Can you work these out from the model? Positions are in its coordinate system, mm. Face numbers are marked on the shaded views. A direction names the side the tool comes from. Round coordinates to 2 decimals unless told otherwise and drop trailing zeros. Loops run counter-clockwise (first coordinate to the right, second up) from the corner with the lowest first, then second, coordinate; pieces in that order, holes last. Notation, with made-up numbers: M 4,12 L 8,12 A13 ccw 8,24 Z; hole C 65.25,-26.5 d8. An arc over 180 degrees is marked long. Return JSON: item names as keys, results as strings.
```python
from build123d import *

# Parameters (mm, degrees)
SKETCH1_W           = 28.2
SKETCH1_H           = 28.2
SKETCH1_R           = 1.25
SKETCH1_R_2         = 10
BOSS_EXTRUDE1_DEPTH = 5
SKETCH1_3_R         = 11
SKETCH1_3_R_2       = 10
BOSS_EXTRUDE2_DEPTH = 14
SKETCH1_4_R         = 11
SKETCH1_4_R_2       = 10
CUT_EXTRUDE1_DEPTH  = 2


with BuildPart() as part:
    # Sketch1 → Boss-Extrude1 (new body)
    with BuildSketch(Plane.XY):
        Rectangle(SKETCH1_W, SKETCH1_H)
        with Locations((-11.5, 11.5)):
            Circle(SKETCH1_R, mode=Mode.SUBTRACT)
        with Locations((11.5, 11.5)):
            Circle(SKETCH1_R, mode=Mode.SUBTRACT)
        with Locations((11.5, -11.5)):
            Circle(SKETCH1_R, mode=Mode.SUBTRACT)
        with Locations((-11.5, -11.5)):
            Circle(SKETCH1_R, mode=Mode.SUBTRACT)
        Circle(SKETCH1_R_2, mode=Mode.SUBTRACT)
    extrude(amount=BOSS_EXTRUDE1_DEPTH)

    # Sketch1_3 → Boss-Extrude2 (add)
    # profile 1 of 3: a face of its own
    with BuildSketch(Plane.XY):
        with BuildLine():
            Line((3.4278273, 11.5), (-3.4278273, 11.5))
            ThreePointArc((-3.4278273, 11.5), (-7.17168294, -9.621172683), (12, 0))
            ThreePointArc((12, 0), (9.621172683, 7.17168294), (3.4278273, 11.5))
        make_face()
        Circle(SKETCH1_3_R, mode=Mode.SUBTRACT)
    # profile 2 of 3: a face of its own
    with BuildSketch(Plane.XY):
        Circle(SKETCH1_3_R)
        Circle(SKETCH1_3_R_2, mode=Mode.SUBTRACT)
    # profile 3 of 3: a face of its own
    with BuildSketch(Plane.XY):
        with BuildLine():
            ThreePointArc((3.4278273, 11.5), (0, 12), (-3.4278273, 11.5))
            Line((-3.4278273, 11.5), (3.4278273, 11.5))
        make_face()
    extrude(amount=BOSS_EXTRUDE2_DEPTH)

    # Sketch1_4 → Cut-Extrude1 (cut)
    with BuildSketch(Plane.XY):
        Circle(SKETCH1_4_R)
        Circle(SKETCH1_4_R_2, mode=Mode.SUBTRACT)
    extrude(amount=CUT_EXTRUDE1_DEPTH, mode=Mode.SUBTRACT)


solid = part.part
```
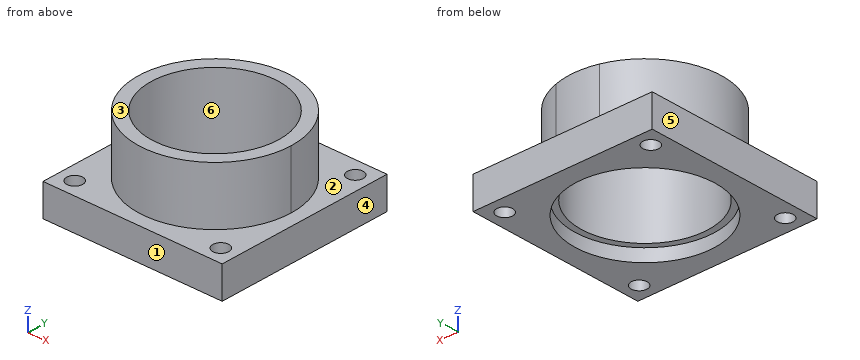
Q1. Suppose I cut it at D-D, the plane y = 4.75. Please give me the cut outline in (x, z).
Results:
{"outline": "M -14.1,0 L -9.92,0 L -9.92,2 L -8.8,2 L -8.8,14 L -11.02,14 L -11.02,5 L -14.1,5 Z; M 8.8,2 L 9.92,2 L 9.92,0 L 14.1,0 L 14.1,5 L 11.02,5 L 11.02,14 L 8.8,14 Z"}
Q2. If I drill on line 1 along Y through (x, z) = (-11.5, 3); line 2 along Y through (x, z) = (-4, 0.75); line 3 along Z through (x, y) = (-1.5, -10.5), over which ranges is the centre line in solid material (lowest first)?
Results:
{"line 1": "y = -14.1 to -12.75, -10.25 to 10.25, 12.75 to 14.1", "line 2": "y = -14.1 to -10.25, 10.25 to 14.1", "line 3": "z = 2 to 14"}
Q3. On a 3-axis mill with a long thin cutter (end or side, diameter ignored), from which of +Z, -Z, +X, -X, +Y, -Y can I reach the whole of each face in a straight line? I mean the marked faces 1 and 2. Say none if no direction works.
Results:
{"face 1": "+Z, -Z, +X, -X, -Y", "face 2": "+Z"}
Q4. I'm going to push flat-ended pins straight in: pin 1 Ø1.5 at (y, z) = (-6.5, 12.5) entering from +X; pin 2 Ø2 at (x, z) = (8, 10) entering from -Y. Where does each tip first touch, or does it pass through?
Results:
{"pin 1": "stops at x = 10.53", "pin 2": "stops at y = -9.75"}
Q5. Thinking about a two-plate mould opening in X: for the marked faces 3, 4, 5 and 6, which applies, pulls with the +X half, pulls with the -X half, needs draft (parallel to the pull), parting line crosses it, or undercut?
Results:
{"face 3": "needs draft", "face 4": "pulls with the +X half", "face 5": "pulls with the -X half", "face 6": "undercut"}
Q6. Suppose I cut it at A-A, the plane x = 0. Please give me the cut outline in (y, z), plus the area to 3 significant figures.
Results:
{"outline": "M -14.1,0 L -11,0 L -11,2 L -10,2 L -10,14 L -12,14 L -12,5 L -14.1,5 Z; M 10,2 L 11,2 L 11,0 L 14.1,0 L 14.1,5 L 12,5 L 12,14 L 10,14 Z", "area": "73.0 mm2"}
Q7. Suppose I cut it at B-B, the plane x = -11.5. Please give me the cut outline in (y, z).
Results:
{"outline": "M -14.1,0 L -12.75,0 L -12.75,5 L -14.1,5 Z; M -10.25,0 L 10.25,0 L 10.25,5 L 3.43,5 L 3.43,14 L -3.43,14 L -3.43,5 L -10.25,5 Z; M 12.75,0 L 14.1,0 L 14.1,5 L 12.75,5 Z"}
